from build123d import *

# Parameters (mm, degrees)
F1_DEPTH = 8
F2_R     = 16.7410714552
F3_DEPTH = 4.8
F4_R     = 18.15
F5_DEPTH = 2
F7_R     = 1.25
F8_DEPTH = 25


# Not quite as in the source:
# - a fillet or chamfer that OpenCascade refuses, or shapes differently, is made with other operations: its cross-section is extruded or revolved along the edge and cut away or added


with BuildPart() as f1:
    # F0 (on Top) → F1 (new body)
    with BuildSketch(Plane.XY):
        with BuildLine():
            ThreePointArc((18.2071917808, -1.2492667675), (18.2392948054, -0.625), (18.25, 0))
            ThreePointArc((18.25, 0), (18.2392948054, 0.625), (18.2071917808, 1.2492667675))
            ThreePointArc((18.2071917808, 1.2492667675), (17, 0), (18.2071917808, -1.2492667675))
        make_face()
        with BuildLine():
            ThreePointArc((18.2071917808, 1.2492667675), (18.2392948054, 0.625), (18.25, 0))
            ThreePointArc((18.25, 0), (18.2392948054, -0.625), (18.2071917808, -1.2492667675))
            ThreePointArc((18.2071917808, -1.2492667675), (19.1186166375, -0.8988910596), (19.5, 0))
            ThreePointArc((19.5, 0), (19.1186166375, 0.8988910596), (18.2071917808, 1.2492667675))
        make_face()
        with BuildLine():
            ThreePointArc((18.2071917808, -1.2492667675), (17, 0), (18.2071917808, 1.2492667675))
            ThreePointArc((18.2071917808, 1.2492667675), (16.8608014683, 6.9839726407), (13.7577937774, 11.9910637718))
            ThreePointArc((13.7577937774, 11.9910637718), (12.0208152802, 12.0208152802), (11.9910637718, 13.7577937774))
            ThreePointArc((11.9910637718, 13.7577937774), (6.9839726407, 16.8608014683), (1.2492667675, 18.2071917808))
            ThreePointArc((1.2492667675, 18.2071917808), (0, 17), (-1.2492667675, 18.2071917808))
            ThreePointArc((-1.2492667675, 18.2071917808), (-6.9839726407, 16.8608014683), (-11.9910637718, 13.7577937774))
            ThreePointArc((-11.9910637718, 13.7577937774), (-11.7418265085, 13.3632051737), (-11.6546987567, 12.9046987567))
            ThreePointArc((-11.6546987567, 12.9046987567), (-12.406636901, 11.7582109076), (-13.7577937774, 11.9910637718))
            ThreePointArc((-13.7577937774, 11.9910637718), (-16.8608014683, 6.9839726407), (-18.2071917808, 1.2492667675))
            ThreePointArc((-18.2071917808, 1.2492667675), (-17.3511089404, 0.8686166375), (-17, 0))
            ThreePointArc((-17, 0), (-17.3511089404, -0.8686166375), (-18.2071917808, -1.2492667675))
            ThreePointArc((-18.2071917808, -1.2492667675), (-16.8608014683, -6.9839726407), (-13.7577937774, -11.9910637718))
            ThreePointArc((-13.7577937774, -11.9910637718), (-12.406636901, -11.7582109076), (-11.6546987567, -12.9046987567))
            ThreePointArc((-11.6546987567, -12.9046987567), (-11.7418265085, -13.3632051737), (-11.9910637718, -13.7577937774))
            ThreePointArc((-11.9910637718, -13.7577937774), (-6.9839726407, -16.8608014683), (-1.2492667675, -18.2071917808))
            ThreePointArc((-1.2492667675, -18.2071917808), (0, -17), (1.2492667675, -18.2071917808))
            ThreePointArc((1.2492667675, -18.2071917808), (6.9839726407, -16.8608014683), (11.9910637718, -13.7577937774))
            ThreePointArc((11.9910637718, -13.7577937774), (12.0208152802, -12.0208152802), (13.7577937774, -11.9910637718))
            ThreePointArc((13.7577937774, -11.9910637718), (16.8608014683, -6.9839726407), (18.2071917808, -1.2492667675))
        make_face()
        with BuildLine():
            ThreePointArc((11.9910637718, 13.7577937774), (12.0208152802, 12.0208152802), (13.7577937774, 11.9910637718))
            ThreePointArc((13.7577937774, 11.9910637718), (12.9046987567, 12.9046987567), (11.9910637718, 13.7577937774))
        make_face()
        with BuildLine():
            ThreePointArc((11.9910637718, 13.7577937774), (12.9046987567, 12.9046987567), (13.7577937774, 11.9910637718))
            ThreePointArc((13.7577937774, 11.9910637718), (14.0511866057, 12.406636901), (14.1546987567, 12.9046987567))
            ThreePointArc((14.1546987567, 12.9046987567), (13.3632051737, 14.0675710048), (11.9910637718, 13.7577937774))
        make_face()
        with BuildLine():
            ThreePointArc((14.1546987567, -12.9046987567), (14.0511866057, -12.406636901), (13.7577937774, -11.9910637718))
            ThreePointArc((13.7577937774, -11.9910637718), (12.9046987567, -12.9046987567), (11.9910637718, -13.7577937774))
            ThreePointArc((11.9910637718, -13.7577937774), (13.3632051737, -14.0675710048), (14.1546987567, -12.9046987567))
        make_face()
        with BuildLine():
            ThreePointArc((11.9910637718, -13.7577937774), (12.9046987567, -12.9046987567), (13.7577937774, -11.9910637718))
            ThreePointArc((13.7577937774, -11.9910637718), (12.0208152802, -12.0208152802), (11.9910637718, -13.7577937774))
        make_face()
        with BuildLine():
            ThreePointArc((-1.2492667675, 18.2071917808), (0, 17), (1.2492667675, 18.2071917808))
            ThreePointArc((1.2492667675, 18.2071917808), (0, 18.25), (-1.2492667675, 18.2071917808))
        make_face()
        with BuildLine():
            ThreePointArc((-1.2492667675, 18.2071917808), (0, 18.25), (1.2492667675, 18.2071917808))
            ThreePointArc((1.2492667675, 18.2071917808), (1.2498166784, 18.2285927509), (1.25, 18.25))
            ThreePointArc((1.25, 18.25), (-0.0214072491, 19.4998166784), (-1.2492667675, 18.2071917808))
        make_face()
        with BuildLine():
            ThreePointArc((1.25, -18.25), (1.2498166784, -18.2285927509), (1.2492667675, -18.2071917808))
            ThreePointArc((1.2492667675, -18.2071917808), (0, -18.25), (-1.2492667675, -18.2071917808))
            ThreePointArc((-1.2492667675, -18.2071917808), (-0.0214072491, -19.4998166784), (1.25, -18.25))
        make_face()
        with BuildLine():
            ThreePointArc((-1.2492667675, -18.2071917808), (0, -18.25), (1.2492667675, -18.2071917808))
            ThreePointArc((1.2492667675, -18.2071917808), (0, -17), (-1.2492667675, -18.2071917808))
        make_face()
        with BuildLine():
            ThreePointArc((-11.6546987567, 12.9046987567), (-11.7418265085, 13.3632051737), (-11.9910637718, 13.7577937774))
            ThreePointArc((-11.9910637718, 13.7577937774), (-12.9046987567, 12.9046987567), (-13.7577937774, 11.9910637718))
            ThreePointArc((-13.7577937774, 11.9910637718), (-12.406636901, 11.7582109076), (-11.6546987567, 12.9046987567))
        make_face()
        with BuildLine():
            ThreePointArc((-13.7577937774, 11.9910637718), (-12.9046987567, 12.9046987567), (-11.9910637718, 13.7577937774))
            ThreePointArc((-11.9910637718, 13.7577937774), (-13.7885822331, 13.7885822331), (-13.7577937774, 11.9910637718))
        make_face()
        with BuildLine():
            ThreePointArc((-13.7577937774, -11.9910637718), (-13.7885822331, -13.7885822331), (-11.9910637718, -13.7577937774))
            ThreePointArc((-11.9910637718, -13.7577937774), (-12.9046987567, -12.9046987567), (-13.7577937774, -11.9910637718))
        make_face()
        with BuildLine():
            ThreePointArc((-13.7577937774, -11.9910637718), (-12.9046987567, -12.9046987567), (-11.9910637718, -13.7577937774))
            ThreePointArc((-11.9910637718, -13.7577937774), (-11.7418265085, -13.3632051737), (-11.6546987567, -12.9046987567))
            ThreePointArc((-11.6546987567, -12.9046987567), (-12.406636901, -11.7582109076), (-13.7577937774, -11.9910637718))
        make_face()
        with BuildLine():
            ThreePointArc((-17, 0), (-17.3511089404, 0.8686166375), (-18.2071917808, 1.2492667675))
            ThreePointArc((-18.2071917808, 1.2492667675), (-18.25, 0), (-18.2071917808, -1.2492667675))
            ThreePointArc((-18.2071917808, -1.2492667675), (-17.3511089404, -0.8686166375), (-17, 0))
        make_face()
        with BuildLine():
            ThreePointArc((-18.2071917808, -1.2492667675), (-18.25, 0), (-18.2071917808, 1.2492667675))
            ThreePointArc((-18.2071917808, 1.2492667675), (-19.5, 0), (-18.2071917808, -1.2492667675))
        make_face()
    extrude(amount=F1_DEPTH)

    # F2 (on face) → F3 (cut)
    with BuildSketch(Plane(origin=(0, 0, 0), x_dir=(1, 0, 0), z_dir=(0, 0, -1))):
        Circle(F2_R)
    extrude(amount=-F3_DEPTH, mode=Mode.SUBTRACT)

    # F4 (on face) → F5 (join)
    with BuildSketch(Plane.XY.offset(8)):
        Circle(F4_R)
    extrude(amount=F5_DEPTH)

    # F6: fillet of radius 5 on 1 edges, made by hand

    # F6_s1 → F6_t2 (revolve, cut)
    with BuildSketch(Plane.XZ):
        with BuildLine():
            ThreePointArc((18.15, 8), (16.3860679775, 9.472135955), (14.15, 10))
            Line((14.15, 10), (18.15, 10))
            Line((18.15, 10), (18.15, 8))
        make_face()
    revolve(axis=Axis((0, 0, 10), (0, 0, 1)), mode=Mode.SUBTRACT)

    # F7 (on face) → F8 (cut)
    with BuildSketch(Plane(origin=(0, 0, 4.8), x_dir=(1, 0, 0), z_dir=(0, 0, -1))):
        Circle(F7_R)
    extrude(amount=-F8_DEPTH, mode=Mode.SUBTRACT)


solid = f1.part
Verification items for the finished model (mm, model axes). A direction names the side the tool comes from. Give positions to 0.01 mm unless a question says otherwise; leave off trailing zeros. Write each loop counter-clockwise with the first axis right and the second up, starting at its lowest first coordinate (ties: lowest second). Pieces come first, ordered by that corner, then holes. Notation, with made-up numbers: M 29.25,18.5 L 62.25,18.5 A19 cw 62.25,26.5 Z; hole C 72.5,-34 d8. An arc over 180 degrees is marked long. Put each result on its own line as item: value. Start each with the question number.
1. Go/stop test with flat-tipped pins: pin 1 Ø1.5 at (x, z) = (-8, 3) entering from +Y; pin 2 Ø6 at (y, z) = (-8, 4.5) entering from +X; pin 3 Ø3 at (x, y) = (-5.5, 11.5) entering from -Z; pin 4 Ø1.5 at (x, y) = (0, 0) entering from -Z. Record where each tip stops, or that it passes through.
2. Section check A-A (x = 0). Record the cut outline in (y, z), and give its area (3 significant figures).
3. Section check C-C (z = 1.75). Record the cut outline in (x, y).
4. Set-up check for faces 1 (the face through (13, -13, 8)), 2 (the face through (0, 3, 4.8)), 3 (the face through (6, -16, 0)): record each of +Z, -Z, +X, -X, +Y, -Y from which the full face is reachable in a straight line by a thin tool's end or side.
5. Scan lines: line 1 along Y through (x, z) = (0, 7.1); line 2 along Z through (x, y) = (-12, -5); line 3 along X through (y, z) = (-15, 2.5). Record each from-to range of solid material in increasing order. Write a range as [from, to].
6. Draft check along Y on faces 4 (the face through (15.968, -5.029, 2.366)), 5 (the face through (7.06, 16.83, 3.94)), 6 (the face through (-19.5, 0, 3.9)). Enter one of: +Y half, -Y half, draft (parallel to the pull), parting line (faces both ways), or undercut.
7. Section check B-B (z = 5.25). Record the cut outline in (x, y), and give its area (3 significant figures).
Answer list:
1. pin 1: y = 16.75
1. pin 2: x = 17.55
1. pin 3: z = 4.8
1. pin 4: through
2. outline: M -19.5,0 L -16.74,0 L -16.74,4.8 L -1.25,4.8 L -1.25,10 L -14.15,10 A5 ccw -18.15,8 L -19.5,8 Z; M 1.25,4.8 L 16.74,4.8 L 16.74,0 L 19.5,0 L 19.5,8 L 18.15,8 A5 ccw 14.15,10 L 1.25,10 Z
2. area: 206 mm2
3. outline: M -18.21,-1.25 A18.25 ccw -13.76,-11.99 A1.25 ccw long -11.99,-13.76 A18.25 ccw -1.25,-18.21 A1.25 ccw long 1.25,-18.21 A18.25 ccw 11.99,-13.76 A1.25 ccw long 13.76,-11.99 A18.25 ccw 18.21,-1.25 A1.25 ccw long 18.21,1.25 A18.25 ccw 13.76,11.99 A1.25 ccw long 11.99,13.76 A18.25 ccw 1.25,18.21 A1.25 ccw long -1.25,18.21 A18.25 ccw -11.99,13.76 A1.25 ccw long -13.76,11.99 A18.25 ccw -18.21,1.25 A1.25 ccw long Z; hole C 0,0 d33.48
4. face 1: +Z
4. face 2: -Z
4. face 3: -Z, +X, -X, +Y, -Y
5. line 1: [-19.5, -1.25], [1.25, 19.5]
5. line 2: [4.8, 10]
5. line 3: [-10.4, -7.43], [7.43, 10.4]
6. face 4: undercut
6. face 5: +Y half
6. face 6: parting line
7. outline: M -18.21,-1.25 A18.25 ccw -13.76,-11.99 A1.25 ccw long -11.99,-13.76 A18.25 ccw -1.25,-18.21 A1.25 ccw long 1.25,-18.21 A18.25 ccw 11.99,-13.76 A1.25 ccw long 13.76,-11.99 A18.25 ccw 18.21,-1.25 A1.25 ccw long 18.21,1.25 A18.25 ccw 13.76,11.99 A1.25 ccw long 11.99,13.76 A18.25 ccw 1.25,18.21 A1.25 ccw long -1.25,18.21 A18.25 ccw -11.99,13.76 A1.25 ccw long -13.76,11.99 A18.25 ccw -18.21,1.25 A1.25 ccw long Z; hole C 0,0 d2.5
7. area: 1,060 mm2
